Model file for the job. Use its own axes, mm. Face numbers are marked on the shaded views. Coordinates: 2 decimals unless noted, no trailing zeros. Order: outer loops, then holes, each group sorted by start corner. A loop starts at its lowest first (then second) coordinate and runs counter-clockwise, first axis right, second up.
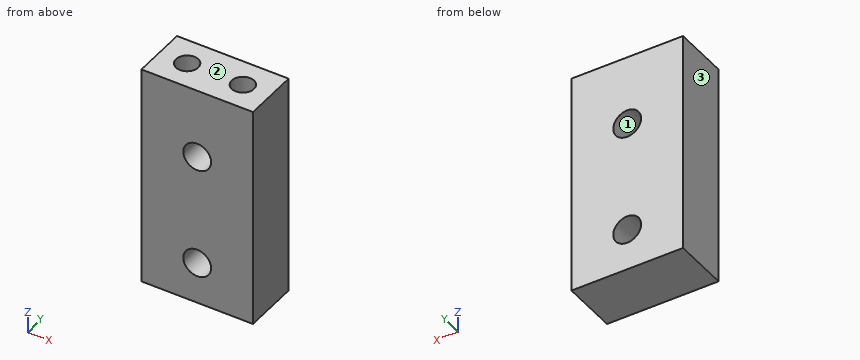
from build123d import *

# Parameters (mm, degrees)
F0_W     = 25.4
F0_H     = 50.8
F0_R     = 3.175
F1_DEPTH = 12.7
F2_R     = 2.54
F3_DEPTH = 25.4


with BuildPart() as f1:
    # F0 (on Front) → F1 (new body)
    with BuildSketch(Plane.XZ):
        Rectangle(F0_W, F0_H)
        with Locations((0, -15.875)):
            Circle(F0_R, mode=Mode.SUBTRACT)
        with Locations((0, 9.525)):
            Circle(F0_R, mode=Mode.SUBTRACT)
    extrude(amount=F1_DEPTH)

    # F2 (on face) → F3 (cut)
    with BuildSketch(Plane.XY.offset(25.4)):
        with Locations((-6.35, -6.35)):
            Circle(F2_R)
        with Locations((6.35, -6.35)):
            Circle(F2_R)
    extrude(amount=-F3_DEPTH, mode=Mode.SUBTRACT)


solid = f1.part
Q1. Cut at C-C, the plane y = -6.35. List the corners of the cut face in (x, z) (3 decimals).
Established:
outline: (-12.7, -25.4) - (12.7, -25.4) - (12.7, 25.4) - (8.89, 25.4) - (8.89, 0) - (3.81, 0) - (3.81, 25.4) - (-3.81, 25.4) - (-3.81, 0) - (-8.89, 0) - (-8.89, 25.4) - (-12.7, 25.4) - close; hole circle Ø6.35 at (0, -15.875); hole circle Ø6.35 at (0, 9.525)
Q2. Cut at D-D, the plane x = 6.35. List the corners of the cut face in (y, z), plus the area to 3 significant figures.
Established:
outline: (-12.7, -25.4) - (0, -25.4) - (0, 25.4) - (-3.81, 25.4) - (-3.81, 0) - (-8.89, 0) - (-8.89, 25.4) - (-12.7, 25.4) - close
area: 516 mm2
Q3. Cut at A-A, the plane x = 0. List the corners of the cut face in (y, z), plus the area to 3 significant figures.
Established:
outline: (-12.7, -25.4) - (0, -25.4) - (0, -19.05) - (-12.7, -19.05) - close; (-12.7, -12.7) - (0, -12.7) - (0, 6.35) - (-12.7, 6.35) - close; (-12.7, 12.7) - (0, 12.7) - (0, 25.4) - (-12.7, 25.4) - close
area: 484 mm2
Q4. Probe line 1 (Z direction, x = 0, y = -8.75); line 2 (X direction, y = -6.5, z = 18); line 3 (X direction, y = -1.5, z = -16). List the from-to ranges inside material, lowest first.
Established:
line 1: z = -25.4 to -19.05, -12.7 to 6.35, 12.7 to 25.4
line 2: x = -12.7 to -8.89, -3.81 to 3.81, 8.89 to 12.7
line 3: x = -12.7 to -3.17, 3.17 to 12.7
Q5. Cut at B-B, the plane z = 7.5. List the corners of the cut face in (x, y).
Established:
outline: (-12.7, -12.7) - (-2.45, -12.7) - (-2.45, 0) - (-12.7, 0) - close; (2.45, -12.7) - (12.7, -12.7) - (12.7, 0) - (2.45, 0) - close; hole circle Ø5.08 at (-6.35, -6.35); hole circle Ø5.08 at (6.35, -6.35)
Q6. Mould opens along X. For the marked faces 1, 2 and 3 say: pulls with the +X half, pulls with the -X half, needs draft (parallel to the pull), parting line crosses it, or undercut.
Established:
face 1: undercut
face 2: needs draft
face 3: pulls with the -X half
Q7. Drop a flat-ended pin along its axis: P1, Ø3, axis at x = 6.35, y = -6.35, coming from the +Z side. Give the stop position or say it passes through.
Established:
P1: stops at z = 0
